from build123d import *

# Parameters (mm, degrees)
SKETCH1_R           = 12.5
BOSS_EXTRUDE1_DEPTH = 10
CUT_EXTRUDE1_REACH  = 98.644
SKETCH2_R           = 2.5
SKETCH2_3_R         = 6
SKETCH2_3_R_2       = 2.5
CUT_EXTRUDE2_DEPTH  = 4
CUT_EXTRUDE4_REACH  = 98.644
SKETCH3_R           = 1.5
SKETCH3_4_R         = 3.5
SKETCH3_4_R_2       = 1.5
CUT_EXTRUDE5_DEPTH  = 5


with BuildPart() as part:
    # Sketch1 → Boss-Extrude1 (new body)
    with BuildSketch(Plane.XY):
        with Locations((0, 75)):
            Circle(SKETCH1_R)
        with BuildLine():
            Line((-39.79776757, 0), (39.79776757, 0))
            Line((39.79776757, 0), (12.5, 75))
            ThreePointArc((12.5, 75), (10.716279715, 68.564834962), (5.87418415, 63.966235431))
            Line((5.87418415, 63.966235431), (25.516287503, 10))
            Line((25.516287503, 10), (-25.516287503, 10))
            Line((-25.516287503, 10), (-5.87418415, 63.966235431))
            ThreePointArc((-5.87418415, 63.966235431), (-10.716279715, 68.564834962), (-12.5, 75))
            Line((-12.5, 75), (-39.79776757, 0))
        make_face()
        with BuildLine():
            Line((-5, 10), (5, 10))
            Line((5, 10), (5, 63.543560763))
            ThreePointArc((5, 63.543560763), (0, 62.5), (-5, 63.543560763))
            Line((-5, 63.543560763), (-5, 10))
        make_face()
    extrude(amount=BOSS_EXTRUDE1_DEPTH)

    # Sketch2 → Cut-Extrude1 (cut, up to next)
    with BuildSketch(Plane.XY.offset(10), mode=Mode.PRIVATE) as cut_extrude1_sk1:
        with Locations((0, 75)):
            Circle(SKETCH2_R)
    cut_extrude1_tool1 = extrude(cut_extrude1_sk1.sketch, amount=-CUT_EXTRUDE1_REACH, mode=Mode.PRIVATE) & part.part
    add(cut_extrude1_tool1.solids().sort_by_distance((0, 75, 10))[0], mode=Mode.SUBTRACT)

    # Sketch2_3 → Cut-Extrude2 (cut)
    with BuildSketch(Plane.XY.offset(10)):
        with Locations((0, 75)):
            Circle(SKETCH2_3_R)
        with Locations((0, 75)):
            Circle(SKETCH2_3_R_2, mode=Mode.SUBTRACT)
    extrude(amount=-CUT_EXTRUDE2_DEPTH, mode=Mode.SUBTRACT)

    # Sketch3 → Cut-Extrude4 (cut, up to next)
    with BuildSketch(Plane.XY.offset(10), mode=Mode.PRIVATE) as cut_extrude4_sk1:
        with Locations((-31.29776757, 5)):
            Circle(SKETCH3_R)
    cut_extrude4_tool1 = extrude(cut_extrude4_sk1.sketch, amount=-CUT_EXTRUDE4_REACH, mode=Mode.PRIVATE) & part.part
    # Sketch3 → Cut-Extrude4 (cut, up to next)
    with BuildSketch(Plane.XY.offset(10), mode=Mode.PRIVATE) as cut_extrude4_sk2:
        with Locations((0, 5)):
            Circle(SKETCH3_R)
    cut_extrude4_tool2 = extrude(cut_extrude4_sk2.sketch, amount=-CUT_EXTRUDE4_REACH, mode=Mode.PRIVATE) & part.part
    # Sketch3 → Cut-Extrude4 (cut, up to next)
    with BuildSketch(Plane.XY.offset(10), mode=Mode.PRIVATE) as cut_extrude4_sk3:
        with Locations((31.29776757, 5)):
            Circle(SKETCH3_R)
    cut_extrude4_tool3 = extrude(cut_extrude4_sk3.sketch, amount=-CUT_EXTRUDE4_REACH, mode=Mode.PRIVATE) & part.part
    # Sketch3 → Cut-Extrude4 (cut, up to next)
    with BuildSketch(Plane.XY.offset(10), mode=Mode.PRIVATE) as cut_extrude4_sk4:
        with Locations((0, 62)):
            Circle(SKETCH3_R)
    cut_extrude4_tool4 = extrude(cut_extrude4_sk4.sketch, amount=-CUT_EXTRUDE4_REACH, mode=Mode.PRIVATE) & part.part
    add(cut_extrude4_tool1.solids().sort_by_distance((-31.297768, 5, 10))[0], mode=Mode.SUBTRACT)
    add(cut_extrude4_tool2.solids().sort_by_distance((0, 5, 10))[0], mode=Mode.SUBTRACT)
    add(cut_extrude4_tool3.solids().sort_by_distance((31.297768, 5, 10))[0], mode=Mode.SUBTRACT)
    add(cut_extrude4_tool4.solids().sort_by_distance((0, 62, 10))[0], mode=Mode.SUBTRACT)

    # Sketch3_4 → Cut-Extrude5 (cut)
    # profile 1 of 4: a face of its own
    with BuildSketch(Plane.XY.offset(10)):
        with Locations((-31.29776757, 5)):
            Circle(SKETCH3_4_R)
        with Locations((-31.29776757, 5)):
            Circle(SKETCH3_4_R_2, mode=Mode.SUBTRACT)
    # profile 2 of 4: a face of its own
    with BuildSketch(Plane.XY.offset(10)):
        with Locations((0, 5)):
            Circle(SKETCH3_4_R)
        with Locations((0, 5)):
            Circle(SKETCH3_4_R_2, mode=Mode.SUBTRACT)
    # profile 3 of 4: a face of its own
    with BuildSketch(Plane.XY.offset(10)):
        with Locations((31.29776757, 5)):
            Circle(SKETCH3_4_R)
        with Locations((31.29776757, 5)):
            Circle(SKETCH3_4_R_2, mode=Mode.SUBTRACT)
    # profile 4 of 4: a face of its own
    with BuildSketch(Plane.XY.offset(10)):
        with Locations((0, 62)):
            Circle(SKETCH3_4_R)
    extrude(amount=-CUT_EXTRUDE5_DEPTH, mode=Mode.SUBTRACT)


solid = part.part
Part model, mm, in its own coordinate system. A direction names the side the tool comes from. Give positions to 0.01 mm unless a question says otherwise; leave off trailing zeros. Order: outer loops, then holes, each group sorted by start corner. A loop starts at its lowest first (then second) coordinate and runs counter-clockwise, first axis right, second up. Notation, with made-up numbers: (-7.75, -14.75) -> (9.25, -14.75) arc R16 ccw to (9.25, 3.25) -> close; hole circle Ø6 at (72, -12.75). An arc over 180 degrees is marked (long way). Use one line per item in the form item = value.
(1) Saw through at A-A (y = 5). Write the cut outline in (x, z), then the cut area to 3 significant figures.
Solution:
outline = (-37.98, 0) -> (-32.8, 0) -> (-32.8, 5) -> (-34.8, 5) -> (-34.8, 10) -> (-37.98, 10) -> close; (-29.8, 0) -> (-1.5, 0) -> (-1.5, 5) -> (-3.5, 5) -> (-3.5, 10) -> (-27.8, 10) -> (-27.8, 5) -> (-29.8, 5) -> close; (1.5, 0) -> (29.8, 0) -> (29.8, 5) -> (27.8, 5) -> (27.8, 10) -> (3.5, 10) -> (3.5, 5) -> (1.5, 5) -> close; (32.8, 0) -> (37.98, 0) -> (37.98, 10) -> (34.8, 10) -> (34.8, 5) -> (32.8, 5) -> close
area = 610 mm²
(2) Flat gauge pins, fed straight in: P1, Ø5, axis at y = 35.5, z = 6, coming from the -X side; P2, Ø5, axis at y = 25.5, z = 7.5, coming from the -X side; P3, Ø3.5, axis at x = -1.5, y = 75, coming from the +Z side; P4, Ø9, axis at x = 31.3, y = 5, coming from the +Z side. Where does each tip first touch, or does it go through?
Solution:
P1 = -27.79
P2 = -31.43
P3 = 6
P4 = 10
(3) Saw through at B-B (z = 7.75). Write the cut outline in (x, y), then the cut area to 3 significant figures.
Solution:
outline = (-39.8, 0) -> (39.8, 0) -> (12.5, 75) arc R12.5 ccw to (-12.5, 75) -> close; hole circle Ø7 at (-31.3, 5); hole (-25.52, 10) -> (-5, 10) -> (-5, 63.54) arc R12.5 cw to (-5.87, 63.97) -> close; hole circle Ø12 at (0, 75); hole circle Ø7 at (0, 5); hole circle Ø7 at (0, 62); hole (5, 10) -> (25.52, 10) -> (5.87, 63.97) arc R12.5 cw to (5, 63.54) -> close; hole circle Ø7 at (31.3, 5)
area = 2,750 mm²
(4) Saw through at D-D (y = 76). Write the cut outline in (x, z).
Solution:
outline = (-12.46, 0) -> (-2.29, 0) -> (-2.29, 6) -> (-5.92, 6) -> (-5.92, 10) -> (-12.46, 10) -> close; (2.29, 0) -> (12.46, 0) -> (12.46, 10) -> (5.92, 10) -> (5.92, 6) -> (2.29, 6) -> close
(5) Pull direction Y, two halves, no side cores. Call faces 1 (the face through (1.615, 1.895, 7.535)), 2 (the face through (0.275, 87.497, 4.93)), 3 (the face through (-1, 35, 10)): +Y half, -Y half, draft (parallel to the pull), parting line (faces both ways), or undercut.
Solution:
face_1 = undercut
face_2 = +Y half
face_3 = draft
(6) Saw through at C-C (x = 0). Write the cut outline in (y, z), then the cut area to 3 significant figures.
Solution:
outline = (0, 0) -> (3.5, 0) -> (3.5, 5) -> (1.5, 5) -> (1.5, 10) -> (0, 10) -> close; (6.5, 0) -> (60.5, 0) -> (60.5, 5) -> (58.5, 5) -> (58.5, 10) -> (8.5, 10) -> (8.5, 5) -> (6.5, 5) -> close; (63.5, 0) -> (72.5, 0) -> (72.5, 6) -> (69, 6) -> (69, 10) -> (65.5, 10) -> (65.5, 5) -> (63.5, 5) -> close; (77.5, 0) -> (87.5, 0) -> (87.5, 10) -> (81, 10) -> (81, 6) -> (77.5, 6) -> close
area = 697 mm²
(7) Drill centre lines: line 1 (Y direction, x = 0, z = 2.75); line 2 (Y direction, x = 0, z = 8.85); line 3 (X direction, y = 30, z = 7). Where is each one in solid material? Low to high. Write a range as from..to.
Solution:
line_1 = 0..3.5, 6.5..60.5, 63.5..72.5, 77.5..87.5
line_2 = 0..1.5, 8.5..58.5, 65.5..69, 81..87.5
line_3 = -28.88..-18.24, -5..5, 18.24..28.88
(8) Tool access for faces 4 (the face through (-25.96, 38.02, 4.93)), 5 (the face through (5, 36, 5)), 6 (the face through (27.8, 5.15, 7.54)): list every direction of +Z, -Z, +X, -X, +Y, -Y with a clear straight run to the whole face (end or side of a thin tool).
Solution:
face_4 = +Z, -Z, -X, +Y
face_5 = +Z, -Z
face_6 = +Z
